Autodesk Inventor part; units mm, degrees
ref_plane "YZ Plane" through (0, 0, 0) normal (1, 0, 0) x (0, 1, 0)
ref_plane "XZ Plane" through (0, 0, 0) normal (0, 1, 0) x (-1, 0, 0)
ref_plane "XY Plane" through (0, 0, 0) normal (0, 0, 1) x (1, 0, 0)
sketch "Sketch1" plane through (0, 0, 0) normal (0, 0, 1) x (1, 0, 0)
  circle A0 centre (0, 0) radius 7.5
  circle A1 centre (4.7555, -31.9787) radius 6.5
  circle A2 centre (-29.46, -40.6707) radius 6.5
  circle A3 centre (-8.4678, -55.1389) radius 6.5
  circle A4 centre (-143.4307, 8.331) radius 7.4
  circle A5 centre (-305.2033, 72.4426) radius 6.5
  circle A6 centre (-140.546, 409.84) radius 6.5
  circle A7 centre (-11.0649, 354.1696) radius 6.5
  circle A8 centre (0, 0) radius 6 construction
  line L0 (5.7316, -1.7744) -> (-2.8867, -29.6128)
  arc A9 (-2.8867, -29.6128) -> (-3.232, -32.4269) centre (4.7555, -31.9787) ccw
  line L1 (-3.232, -32.4269) -> (-1.978, -54.7747)
  line L2 (-11.0352, -61.1103) -> (-307.7707, 66.4712)
  line L3 (-311.0448, 75.2934) -> (-146.3875, 412.6908)
  line L4 (-137.9786, 415.8114) -> (-8.4975, 360.141)
  line L5 (-5.0935, 351.6021) -> (-60.7594, 222.1316)
  line L6 (-5.6477, 2.0256) -> (-21.9297, -43.3715)
  arc A10 (-32.5665, -48.0429) -> (-21.9297, -43.3715) centre (-29.46, -40.6707) ccw
  line L7 (-32.5665, -48.0429) -> (-146.8867, 0.1294)
  arc A11 (-151.607, 11.8464) -> (-146.8867, 0.1294) centre (-143.4307, 8.331) ccw
  line L8 (-151.607, 11.8464) -> (-67.3996, 207.7001)
  arc A12 (-311.0448, 75.2934) -> (-307.7707, 66.4712) centre (-305.2033, 72.4426) ccw
  arc A13 (-137.9786, 415.8114) -> (-146.3875, 412.6908) centre (-140.546, 409.84) ccw
  arc A14 (-5.0935, 351.6021) -> (-8.4975, 360.141) centre (-11.0649, 354.1696) ccw
  arc A15 (5.7316, -1.7744) -> (-5.6477, 2.0256) centre (0, 0) ccw
  arc A16 (-11.0352, -61.1103) -> (-1.978, -54.7747) centre (-8.4678, -55.1389) ccw
  line L9 (-59.3813, 221.5391) -> (-3.7154, 351.0096)
  arc A17 (-3.7154, 351.0096) -> (-7.905, 361.519) centre (-11.0649, 354.1696) ccw
  line L10 (-7.905, 361.519) -> (-137.3861, 417.1895)
  arc A18 (-137.3861, 417.1895) -> (-147.7355, 413.3486) centre (-140.546, 409.84) ccw
  line L11 (-147.7355, 413.3486) -> (-312.3928, 75.9513)
  arc A19 (-312.3928, 75.9513) -> (-308.3632, 65.0932) centre (-305.2033, 72.4426) ccw
  line L12 (-308.3632, 65.0932) -> (-11.6277, -62.4884)
  arc A20 (-11.6277, -62.4884) -> (-0.4804, -54.6907) centre (-8.4678, -55.1389) ccw
  line L13 (-0.4804, -54.6907) -> (-1.7343, -32.3428)
  arc A21 (-1.4538, -30.0564) -> (-1.7343, -32.3428) centre (4.7555, -31.9787) ccw
  line L14 (-1.4538, -30.0564) -> (7.1645, -2.218)
  arc A22 (7.1645, -2.218) -> (-7.0597, 2.532) centre (0, 0) ccw
  line L15 (-7.0597, 2.532) -> (-23.3416, -42.8651)
  arc A23 (-31.9841, -46.6606) -> (-23.3416, -42.8651) centre (-29.46, -40.6707) ccw
  line L16 (-31.9841, -46.6606) -> (-146.3042, 1.5117)
  arc A24 (-150.2289, 11.2539) -> (-146.3042, 1.5117) centre (-143.4307, 8.331) ccw
  line L17 (-150.2289, 11.2539) -> (-66.0216, 207.1076)
  line L18 (-67.3996, 207.7001) -> (-66.0216, 207.1076)
  line L19 (-60.7594, 222.1316) -> (-59.3813, 221.5391)
  point P0 (0, 0)
  dimension "d0" = 12
  dimension "d1" = 1.5
  dimension "d2" = 1.5
  dimension "d3" = 1.5
  dimension "d4" = 1.5
extrude "Extrusion1" add sketch "Sketch1" along normal blind 6 contours A0 L0 A15 L6 | A0 L6 A10 L7 A11 L8 L18 L17 A4 L16 A2 L15 | L14 A1 L13 A20 L12 A19 L11 A18 L10 A17 L9 L19 L5 A7 L4 A6 L3 A5 L2 A3 L1 A9 L0 A0 picked at (-6.7626, -0.2729)
properties part number "BeltRight" material "Rubber"
Model file for the job. Use its own axes, mm. A direction names the side the tool comes from. Coordinates: 2 decimals unless noted, no trailing zeros. Write each loop counter-clockwise with the first axis right and the second up, starting at its lowest first coordinate (ties: lowest second). Pieces come first, ordered by that corner, then holes. Notation, with made-up numbers: (13.5, -0.75) - (68.5, -0.75) arc R14 cw to (68.5, 11.25) - close; hole circle Ø1 at (21.25, 16.25). An arc over 180 degrees is marked (long way). Write each question's results on one line, items separated by ' | '. Start each with the question number.
1) 3-axis set-ups, long thin cutter, end or side, ignore diameter. For faces 5 (the face through (-228.912, 247.012, 2.958)), 6 (the face through (-157.33, 1.79, 2.96)), 7 (the face through (-108.715, 107.81, 2.958)): which of +Z, -Z, +X, -X, +Y, -Y reach the whole face in a straight line?
2) Probe line 1 along Y through (x, z) = (-33, 4.75); line 2 along X through (y, z) = (384, 3.2); line 3 along X through (y, z) = (-28.5, 4.8). List the from-to ranges inside material, lowest first. Write a range as from..to.
3) Mould opens along Y. For faces 1 (the face through (-13.675, -20.355, 2.958)), 2 (the face through (-162.073, 2.195, 2.958)), 3 (the face through (-15.087, -19.849, 2.958)), 4 (the face through (-71.739, 388.965, 2.958)) say: pulls with the +Y half, pulls with the -Y half, needs draft (parallel to the pull), parting line crosses it, or undercut.
4) Cut at B-B (x = -105). Write the cut outline in (y, z).
5) Flat gauge pins, fed straight in: P1, Ø1, axis at y = 20, z = 2.5, coming from the +X side; P2, Ø1.5, axis at y = 359, z = 5, coming from the -X side; P3, Ø1.5, axis at x = -165.5, z = 3.5, coming from the +Y side. Where does each tip first touch, or does it go through?
6) Cut at A-A (y = 173). Write the cut outline in (x, z), then the cut area to 3 significant figures.
7) Cut at C-C (x = -212.5). Write the cut outline in (y, z).
Returned:
1) face 5: +Z, -Z, -X, +Y | face 6: +Z, -Z | face 7: +Z, -Z, +X
2) line 1: -53.3..-51.67, -47.86..-46.23, 282.9..286.7, 370.68..372.31 | line 2: -162.06..-160.39, -63.99..-60.19 | line 3: -90.68..-86.88, -78.94..-75.08, -18.19..-16.6, -2.54..-0.97
3) face 1: undercut | face 2: pulls with the -Y half | face 3: undercut | face 4: pulls with the +Y half
4) outline: (-22.34, 0) - (-20.71, 0) - (-20.71, 6) - (-22.34, 6) - close; (-17.52, 0) - (-15.89, 0) - (-15.89, 6) - (-17.52, 6) - close; (116.45, 0) - (120.25, 0) - (120.25, 6) - (116.45, 6) - close; (401.63, 0) - (403.27, 0) - (403.27, 6) - (401.63, 6) - close
5) P1: x = -146.25 | P2: x = -174.62 | P3: y = 378.48
6) outline: (-265.03, 0) - (-263.36, 0) - (-263.36, 6) - (-265.03, 6) - close; (-82.32, 0) - (-80.69, 0) - (-80.69, 6) - (-82.32, 6) - close | area: 19.8 mm^2
7) outline: (23.88, 0) - (25.51, 0) - (25.51, 6) - (23.88, 6) - close; (277.22, 0) - (280.64, 0) - (280.64, 6) - (277.22, 6) - close
